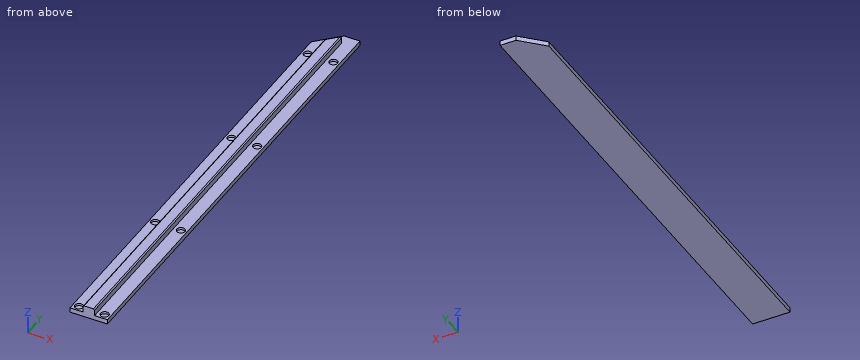
Autodesk Fusion 360 part; units mm, degrees
sketch "3D-printed conduit top outline" plane through (0, 0, 0) normal (0, 1, 0) x (1, 0, 0)
  line L0 (0, 0) -> (16, 0)
  line L1 (16, 0) -> (16, -2)
  line L2 (16, -2) -> (0, -2)
  line L3 (0, -2) -> (0, 0)
  dimension "d7" = 16
  dimension "d8" = 2
extrude "Extrude1" add sketch "3D-printed conduit top outline" along normal blind 201
sketch "Magnet holes" plane through (0, 0, 2) normal (0, 0, 1) x (-1, 0, 0)
  line L0 (0, 0) -> (-16, 0)
  line L1 (-16, 0) -> (-16, -201)
  line L2 (-16, -201) -> (0, -201)
  line L3 (0, -201) -> (0, 0)
  circle A0 centre (-2.5, -2.5) radius 2.5
  circle A1 centre (-13.5, -2.5) radius 2.5
  circle A2 centre (-2.5, -2.5) radius 1.75
  circle A3 centre (-13.5, -2.5) radius 1.75
  circle A4 centre (-2.5, -63.1667) radius 1.75
  circle A5 centre (-2.5, -63.1667) radius 2.5
  circle A6 centre (-13.5, -63.1667) radius 2.5
  circle A7 centre (-13.5, -63.1667) radius 1.75
  circle A8 centre (-2.5, -123.8333) radius 1.75
  circle A9 centre (-2.5, -123.8333) radius 2.5
  circle A10 centre (-13.5, -123.8333) radius 2.5
  circle A11 centre (-13.5, -123.8333) radius 1.75
  circle A12 centre (-2.5, -184.5) radius 1.75
  circle A13 centre (-2.5, -184.5) radius 2.5
  circle A14 centre (-13.5, -184.5) radius 2.5
  circle A15 centre (-13.5, -184.5) radius 1.75
  dimension "d11" = 5
  dimension "d12" = 5
  dimension "d13" = 3.5
  dimension "d14" = 3.5
  dimension "d17" = 0
  dimension "d18" = -182
extrude "Extrude2" cut sketch "Magnet holes" against normal blind 1 contours A2 | A3 | A4 | A7 | A8 | A11 | A12 | A15
sketch "Support rib" plane through (0, 0, 2) normal (0, 0, 1) x (-1, 0, 0)
  line L0 (0, 0) -> (-16, 0)
  line L1 (-16, 0) -> (-16, -201)
  line L2 (-16, -201) -> (0, -201)
  line L3 (0, -201) -> (0, 0)
  circle A0 centre (-13.5, -184.5) radius 1.75
  circle A1 centre (-13.5, -63.1667) radius 1.75
  circle A2 centre (-2.5, -2.5) radius 1.75
  circle A3 centre (-2.5, -123.8333) radius 1.75
  circle A4 centre (-2.5, -184.5) radius 1.75
  circle A5 centre (-2.5, -63.1667) radius 1.75
  circle A6 centre (-13.5, -2.5) radius 1.75
  circle A7 centre (-13.5, -123.8333) radius 1.75
  line L4 (-5.5, 0) -> (-10.5, 0)
  line L5 (-10.5, 0) -> (-10.5, -201)
  line L6 (-10.5, -201) -> (-5.5, -201)
  line L7 (-5.5, -201) -> (-5.5, 0)
  dimension "d23" = 5
  dimension "d24" = 5.5
  dimension "d25" = 5.5
extrude "Extrude3" add sketch "Support rib" along normal blind 3 contours L0 L2 L4 L5 L6 L7
chamfer "Chamfer1" distance 0.5 angle 45 2 edges at (5.5, 100.5, 5) (10.5, 100.5, 5)
sketch "End chamfer" plane through (0, 0, 2) normal (0, 0, 1) x (-1, 0, 0)
  line L0 (-10.5, -201) -> (-10.5, 0)
  line L1 (-10.5, 0) -> (-16, 0)
  line L2 (-16, 0) -> (-16, -201)
  line L3 (-16, -201) -> (-10.5, -201)
  circle A0 centre (-13.5, -123.8333) radius 1.75
  circle A1 centre (-13.5, -2.5) radius 1.75
  circle A2 centre (-13.5, -63.1667) radius 1.75
  circle A3 centre (-13.5, -184.5) radius 1.75
  line L4 (0, -191.828) -> (-9.172, -201)
  line L5 (0, 0) -> (0, -201)
  line L6 (-14.8289, -201) -> (0, -186.1711)
  line L7 (0, -191.828) -> (0, -201)
  line L8 (0, -201) -> (-9.172, -201)
  line L9 (-9.172, -201) -> (-14.8289, -201)
  line L10 (0, -191.828) -> (0, -186.1711)
  dimension "d30" = 6.828
  dimension "d31" = 135
  dimension "d32" = 4
extrude "Extrude4" cut sketch "End chamfer" along normal blind 3 and the other way blind 2 contours L4 L5 L7 L8
extrude "Extrude5" cut sketch "End chamfer" along normal blind 3 contours L0 L3 L6 L9 | L0 L4 L5 L6 L9 L10
equation "conduit_length = 201 mm"
equation "conduit_width = 16 mm"
equation "conduit_wall_thickness = 2 mm"
equation "magnet_diameter = 3 mm"
equation "magnet_height = 1 mm"
equation "d7 = conduit_width"
equation "d8 = conduit_wall_thickness"
equation "d9 = conduit_length"
equation "d11 = magnet_diameter + 2 mm"
equation "d12 = magnet_diameter + 2 mm"
equation "d13 = magnet_diameter + 0.5 mm"
equation "d14 = magnet_diameter + 0.5 mm"
equation "d18 = -conduit_length + ( magnet_diameter + 2 mm ) + 14 mm"
equation "rib_width = 5 mm"
equation "rib_height = 3 mm"
equation "d23 = rib_width"
equation "d24 = ( conduit_width - rib_width ) / 2"
equation "d26 = rib_height"
equation "rib_chamfer = 0.5 mm"
equation "d29 = rib_chamfer"
equation "d32 = 2 * conduit_wall_thickness"
equation "d33 = rib_height"
equation "d35 = conduit_wall_thickness"
equation "d37 = rib_height"
Build history of the part. All positions in model axes, mm. Give positions to 0.01 mm unless a question says otherwise; leave off trailing zeros. Write each loop counter-clockwise with the first axis right and the second up, starting at its lowest first coordinate (ties: lowest second). Pieces come first, ordered by that corner, then holes. Notation, with made-up numbers: (63, -5.75) - (110, -5.75) arc R26 cw to (110, 14.25) - close; hole circle Ø10 at (-24, 46). An arc over 180 degrees is marked (long way). Use one line per item in the form item = value. Start each with the question number.
1. Band-saw the part on A-A on y = 128. Write the cut outline in (x, z), plus the area to 4 significant figures.
2. Band-saw the part on B-B on x = 13.5. Write the cut outline in (y, z), plus the area to 3 significant figures.
3. Band-saw the part on D-D on z = 3.1. Write the cut outline in (x, y), plus the area to 3 significant figures.
4. Drop flat-ended pins along their axis: pin 1 Ø1.7 at (x, y) = (12.5, 63.5) entering from +Z; pin 2 Ø3 at (x, y) = (7, 103.5) entering from -Z; pin 3 Ø2 at (x, y) = (2.5, 2.5) entering from +Z. Give the stop position or say it passes through.
5. Probe line 1 (X direction, y = 2.5, z = 1.3); line 2 (Y direction, x = 13.5, z = 1.3); line 3 (Y direction, x = 2.5, z = 1.4). List the from-to ranges inside material, lowest first. Write a range as [from, to].
6. Band-saw the part on C-C on y = 184.5. Write the cut outline in (x, z), plus the area to 4 significant figures.
Conclusion:
q1.outline = (0, 0) - (16, 0) - (16, 2) - (10.5, 2) - (10.5, 4.5) - (10, 5) - (6, 5) - (5.5, 4.5) - (5.5, 2) - (0, 2) - close
q1.area = 46.75 mm²
q2.outline = (0, 0) - (201, 0) - (201, 2) - (186.25, 2) - (186.25, 1) - (182.75, 1) - (182.75, 2) - (125.58, 2) - (125.58, 1) - (122.08, 1) - (122.08, 2) - (64.92, 2) - (64.92, 1) - (61.42, 1) - (61.42, 2) - (4.25, 2) - (4.25, 1) - (0.75, 1) - (0.75, 2) - (0, 2) - close
q2.area = 388 mm²
q3.outline = (5.5, 0) - (10.5, 0) - (10.5, 196.67) - (5.5, 191.67) - close
q3.area = 971 mm²
q4.pin_1 = 2
q4.pin_2 = 0
q4.pin_3 = 1
q5.line_1 = [0, 0.75], [4.25, 11.75], [15.25, 16]
q5.line_2 = [0, 0.75], [4.25, 61.42], [64.92, 122.08], [125.58, 182.75], [186.25, 201]
q5.line_3 = [0, 0.75], [4.25, 61.42], [64.92, 122.08], [125.58, 182.75], [186.25, 194.33]
q6.outline = (0, 0) - (16, 0) - (16, 2) - (15.25, 2) - (15.25, 1) - (11.75, 1) - (11.75, 2) - (10.5, 2) - (10.5, 4.5) - (10, 5) - (6, 5) - (5.5, 4.5) - (5.5, 2) - (4.25, 2) - (4.25, 1) - (0.75, 1) - (0.75, 2) - (0, 2) - close
q6.area = 39.75 mm²
